from build123d import *

# Parameters (mm, degrees)
SWEEP_THIN6_PROFILE_R   = 9.125
SWEEP_THIN6_PROFILE_R_2 = 6.235


with BuildPart() as part:
    # Sweep-Thin6: sweep along a path in Sketch78
    with BuildLine(Plane.XY) as sweep_thin6_path:
        Line((0, 0), (0, 53.104143086))
        ThreePointArc((0, 53.104143086), (2.874997927, 60.045002073), (9.815856914, 62.92))
        Line((9.815856914, 62.92), (62.92, 62.92))
    # Sweep-Thin6 profile (on start of the path) → Sweep-Thin6 (sweep)
    with BuildSketch(Plane.ZX):
        Circle(SWEEP_THIN6_PROFILE_R)
        Circle(SWEEP_THIN6_PROFILE_R_2, mode=Mode.SUBTRACT)
    sweep(path=sweep_thin6_path.line)


solid = part.part
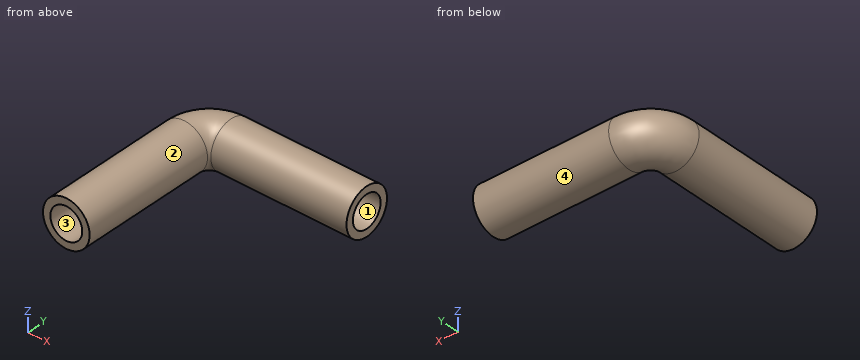
For this review, take the finished solid that the model builds, in its own axes (mm). Face numbers are marked on the shaded views. A direction names the side the tool comes from. Coordinates: 2 decimals unless noted, no trailing zeros. Loops run counter-clockwise (first coordinate to the right, second up) from the corner with the lowest first, then second, coordinate; pieces in that order, holes last. Notation, with made-up numbers: (14.25, -16.75) - (20.25, -16.75) arc R24 ccw to (20.25, 4.25) - close; hole circle Ø10 at (64, 83). An arc over 180 degrees is marked (long way). Return JSON: item names as keys, results as strings.
Item 1: Mouldability with a two-part tool opening along Z and no side actions: class the marked faces 3 and 4 as pulls with the +Z half, pulls with the -Z half, needs draft (parallel to the pull), parting line crosses it, or undercut.
Determined:
{"face 3": "undercut", "face 4": "parting line crosses it"}
Item 2: Take a section at D-D (z = 7.25). Give the boundary of the cut face in (x, y).
Determined:
{"outline": "(-5.54, 0) - (5.54, 0) - (5.54, 53.1) arc R4.27 cw to (9.82, 57.38) - (62.92, 57.38) - (62.92, 68.46) - (9.82, 68.46) arc R15.36 ccw to (-5.54, 53.1) - close"}
Item 3: Take a section at A-A (z = 0). Give the boundary of the cut face in (x, y) (3 decimals).
Determined:
{"outline": "(-9.125, 0) - (-6.235, 0) - (-6.235, 53.104) arc R16.051 cw to (9.816, 69.155) - (62.92, 69.155) - (62.92, 72.045) - (9.816, 72.045) arc R18.941 ccw to (-9.125, 53.104) - close; (6.235, 0) - (9.125, 0) - (9.125, 53.104) arc R0.691 cw to (9.816, 53.795) - (62.92, 53.795) - (62.92, 56.685) - (9.816, 56.685) arc R3.581 ccw to (6.235, 53.104) - close"}
Item 4: Take a section at B-B (x = 48). Give the boundary of the cut face in (y, z) (3 decimals), then the cut area to 3 significant figures.
Determined:
{"outline": "circle Ø18.25 at (62.92, 0); hole circle Ø12.47 at (62.92, 0)", "area": "139 mm2"}
Item 5: For the marked faces 1 and 2, list the 3-axis set-ups (+Z, -Z, +X, -X, +Y, -Y) from which the entire face can be reached by the end or side of a thin tool; tool diameter is ignored.
Determined:
{"face 1": "+X", "face 2": "-Y"}
Item 6: Take a section at C-C (y = 6). Give the boundary of the cut face in (x, z) (3 decimals), then the cut area to 3 significant figures.
Determined:
{"outline": "circle Ø18.25 at (0, 0); hole circle Ø12.47 at (0, 0)", "area": "139 mm2"}
Item 7: Insertion check: pin 1 (10 mm diameter, centred on x = 10, y = 37.5, fed in from -Z); pin 2 (2 mm diameter, centred on x = 1, y = 36, fed in from +Z) (3 decimals); pin 3 (3 mm diameter, centred on y = 22, z = 5.5, fed in from -X); pin 4 (2 mm diameter, centred on x = 40, z = -2, fed in from -Y). Each pin has a flat end and moves straight along its axis. Give the tip position at first contact, or say it passes through.
Determined:
{"pin 1": "stops at z = -7.63", "pin 2": "stops at z = 9.125", "pin 3": "stops at x = -8.2", "pin 4": "stops at y = 53.85"}
Item 8: For line 1 (Z direction, x = 35, y = 62.92) (3 decimals); line 2 (Y direction, x = 59.5, z = 0) (3 decimals); line 3 (Y direction, x = 59, z = -0.25), list the stretches that pass through material, from the lowest coordinate up.
Determined:
{"line 1": "z = -9.125 to -6.235, 6.235 to 9.125", "line 2": "y = 53.795 to 56.685, 69.155 to 72.045", "line 3": "y = 53.8 to 56.69, 69.15 to 72.04"}
